Part model, mm, in its own coordinate system. A direction names the side the tool comes from. Give positions to 0.01 mm unless a question says otherwise; leave off trailing zeros. Loops run counter-clockwise (first coordinate to the right, second up) from the corner with the lowest first, then second, coordinate; pieces in that order, holes last. Notation, with made-up numbers: M 54.5,-12.75 L 113.5,-12.75 A21 cw 113.5,-5.75 Z; hole C -4,80.5 d11. An arc over 180 degrees is marked long. Put each result on its own line as item: value. Start each with the question number.
```python
from build123d import *

# Parameters (mm, degrees)
F0_W     = 15.6
F0_H     = 9.6
F1_DEPTH = 7.8
F2_R     = 2.45
F2_R_2   = 1.65
F3_DEPTH = 1.7
F5_DEPTH = 2


# Not quite as in the source:
# - a feature names something its author has since deleted; it is built from what else it names


with BuildPart() as f1:
    # F0 (on Front) → F1 (new body)
    with BuildSketch(Plane.XZ):
        with Locations((7.5497636572, 4.7150965011)):
            Rectangle(F0_W, F0_H)
        with BuildLine():
            Line((10.5497636572, 6.6150965011), (10.5497636572, 5.6150965011))
            Line((10.5497636572, 5.6150965011), (10.5497636572, 4.6150965011))
            Line((10.5497636572, 4.6150965011), (10.3781907819, 4.6150965011))
            ThreePointArc((10.3781907819, 4.6150965011), (9.6710840007, 3.4937761575), (8.5497636572, 2.7866693764))
            Line((8.5497636572, 2.7866693764), (8.5497636572, 2.6150965011))
            Line((8.5497636572, 2.6150965011), (7.5497636572, 2.6150965011))
            Line((7.5497636572, 2.6150965011), (6.5497636572, 2.6150965011))
            Line((6.5497636572, 2.6150965011), (6.5497636572, 2.7866693764))
            ThreePointArc((6.5497636572, 2.7866693764), (5.4284433136, 3.4937761575), (4.7213365324, 4.6150965011))
            Line((4.7213365324, 4.6150965011), (4.5497636572, 4.6150965011))
            Line((4.5497636572, 4.6150965011), (4.5497636572, 5.6150965067))
            Line((4.5497636572, 5.6150965067), (4.5497636572, 6.6150965011))
            Line((4.5497636572, 6.6150965011), (4.7213365324, 6.6150965011))
            ThreePointArc((4.7213365324, 6.6150965011), (5.4284433136, 7.7364168447), (6.5497636572, 8.4435236258))
            Line((6.5497636572, 8.4435236258), (6.5497636572, 8.6150965011))
            Line((6.5497636572, 8.6150965011), (7.5497636572, 8.6150965011))
            Line((7.5497636572, 8.6150965011), (8.5497636572, 8.6150965011))
            Line((8.5497636572, 8.6150965011), (8.5497636572, 8.4435236258))
            ThreePointArc((8.5497636572, 8.4435236258), (9.6710840007, 7.7364168447), (10.3781907819, 6.6150965011))
            Line((10.3781907819, 6.6150965011), (10.5497636572, 6.6150965011))
        make_face(mode=Mode.SUBTRACT)
        with BuildLine():
            ThreePointArc((8.5497636572, 2.7866693764), (9.6710840007, 3.4937761575), (10.3781907819, 4.6150965011))
            Line((10.3781907819, 4.6150965011), (8.5497636572, 4.6150965011))
            Line((8.5497636572, 4.6150965011), (8.5497636572, 2.7866693764))
        make_face()
        with BuildLine():
            Line((8.5497636572, 6.6150965011), (10.3781907819, 6.6150965011))
            ThreePointArc((10.3781907819, 6.6150965011), (9.6710840007, 7.7364168447), (8.5497636572, 8.4435236258))
            Line((8.5497636572, 8.4435236258), (8.5497636572, 6.6150965011))
        make_face()
        with BuildLine():
            Line((4.7213365324, 6.6150965011), (6.5497636572, 6.6150965011))
            Line((6.5497636572, 6.6150965011), (6.5497636572, 8.4435236258))
            ThreePointArc((6.5497636572, 8.4435236258), (5.4284433136, 7.7364168447), (4.7213365324, 6.6150965011))
        make_face()
        with BuildLine():
            Line((6.5497636572, 2.7866693764), (6.5497636572, 4.6150965011))
            Line((6.5497636572, 4.6150965011), (4.7213365324, 4.6150965011))
            ThreePointArc((4.7213365324, 4.6150965011), (5.4284433136, 3.4937761575), (6.5497636572, 2.7866693764))
        make_face()
        with BuildLine():
            Line((10.5497636572, 4.6150965011), (10.5497636572, 5.6150965011))
            ThreePointArc((10.5497636572, 5.6150965011), (10.5065593361, 5.1077905649), (10.3781907819, 4.6150965011))
            Line((10.3781907819, 4.6150965011), (10.5497636572, 4.6150965011))
        make_face()
        with BuildLine():
            ThreePointArc((10.3781907819, 6.6150965011), (10.5065593361, 6.1224024373), (10.5497636572, 5.6150965011))
            Line((10.5497636572, 5.6150965011), (10.5497636572, 6.6150965011))
            Line((10.5497636572, 6.6150965011), (10.3781907819, 6.6150965011))
        make_face()
        with BuildLine():
            ThreePointArc((7.5497636572, 8.6150965011), (8.0570695933, 8.5718921801), (8.5497636572, 8.4435236258))
            Line((8.5497636572, 8.4435236258), (8.5497636572, 8.6150965011))
            Line((8.5497636572, 8.6150965011), (7.5497636572, 8.6150965011))
        make_face()
        with BuildLine():
            ThreePointArc((6.5497636572, 8.4435236258), (7.042457721, 8.5718921801), (7.5497636572, 8.6150965011))
            Line((7.5497636572, 8.6150965011), (6.5497636572, 8.6150965011))
            Line((6.5497636572, 8.6150965011), (6.5497636572, 8.4435236258))
        make_face()
        with BuildLine():
            ThreePointArc((4.5497636572, 5.6150965067), (4.5929679787, 6.12240244), (4.7213365324, 6.6150965011))
            Line((4.7213365324, 6.6150965011), (4.5497636572, 6.6150965011))
            Line((4.5497636572, 6.6150965011), (4.5497636572, 5.6150965067))
        make_face()
        with BuildLine():
            Line((4.5497636572, 4.6150965011), (4.7213365324, 4.6150965011))
            ThreePointArc((4.7213365324, 4.6150965011), (4.5929679777, 5.1077905677), (4.5497636572, 5.6150965067))
            Line((4.5497636572, 5.6150965067), (4.5497636572, 4.6150965011))
        make_face()
        with BuildLine():
            Line((6.5497636572, 2.6150965011), (7.5497636572, 2.6150965011))
            ThreePointArc((7.5497636572, 2.6150965011), (7.042457721, 2.6583008221), (6.5497636572, 2.7866693764))
            Line((6.5497636572, 2.7866693764), (6.5497636572, 2.6150965011))
        make_face()
        with BuildLine():
            Line((8.5497636572, 2.6150965011), (8.5497636572, 2.7866693764))
            ThreePointArc((8.5497636572, 2.7866693764), (8.0570695933, 2.6583008221), (7.5497636572, 2.6150965011))
            Line((7.5497636572, 2.6150965011), (8.5497636572, 2.6150965011))
        make_face()
    extrude(amount=F1_DEPTH)

    # F2 (on face) → F3 (join)
    with BuildSketch(Plane.XY.offset(9.5150965011)):
        with Locations((3.7997636572, -3.9)):
            Circle(F2_R)
        with Locations((3.7997636572, -3.9)):
            Circle(F2_R_2, mode=Mode.SUBTRACT)
        with Locations((11.2997636572, -3.9)):
            Circle(F2_R)
        with Locations((11.2997636572, -3.9)):
            Circle(F2_R_2, mode=Mode.SUBTRACT)
    extrude(amount=F3_DEPTH)

    # F4 (on face) → F5 (cut)
    with BuildSketch(Plane(origin=(0, 0, -0.0849034989), x_dir=(1, 0, 0), z_dir=(0, 0, -1))):
        Polygon((1.3497636572, 6.2), (1.3497636572, 3.9), (1.3497636572, 1.6), (7.5497636572, 1.6), (13.7497636572, 1.6), (13.7497636572, 3.9), (13.7497636572, 6.2), (7.5497636572, 6.2), align=None)
    extrude(amount=-F5_DEPTH, mode=Mode.SUBTRACT)


solid = f1.part
```
1) Which spindle directions (+Z, -Z, +X, -X, +Y, -Y) get a long thin tool onto all of the face, cutting with end or side? Do faces 4 (the flat face through (15.35, -4, 5)), 5 (the flat face through (11, -4, 9.515)), 6 (the flat face through (7, -4, 1.915)), 7 (the flat face through (9, -4, 6.615)). Say none if no direction does.
2) Mould opens along Y. For faces 1 (the flat face through (6.55, -4, 4)), 2 (the flat face through (4, -4, 9.515)), 3 (the flat face through (9, -7.8, 4)) say: +Y half, -Y half, draft (parallel to the pull), parting line (faces both ways), or undercut.
3) Wall check: L1, parallel to X at y = -7.5, z = 8; L2, parallel to Z at x = 6, y = -5.75; L3, parallel to Z at x = 5.75, y = -1. Give the ranges that are in metal, low to high.
4) Band-saw the part on A-A on z = 7. Give the cut face in (x, y), then the cut area to 3 significant figures.
5) Band-saw the part on B-B on y = -1. Give the cut face in (x, z), then the cut area to 3 significant figures.
6) Band-saw the part on D-D on x = 6. Give the cut face in (y, z), then the cut area to 3 significant figures.
7) Pin check, flat tips, straight feed: pin 1 Ø2 at (x, z) = (7.5, 3.5) entering from +Y; pin 2 Ø1.5 at (x, y) = (5.5, -5) entering from -Z; pin 3 Ø1 at (x, y) = (12, -4) entering from +Z. Stop position of each tip, or through.
8) Band-saw the part on C-C on z = 10.75. Give the cut face in (x, y), then the cut area to 3 significant figures.
Evaluation:
1. face 4: +Z, -Z, +X, +Y, -Y
1. face 5: +Z
1. face 6: -Z
1. face 7: +Y, -Y
2. face 1: draft
2. face 2: undercut
2. face 3: -Y half
3. L1: -0.25 to 6.55, 8.55 to 15.35
3. L2: 1.92 to 4.62, 6.62 to 9.52
3. L3: -0.08 to 4.62, 6.62 to 9.52
4. outline: M -0.25,-7.8 L 6.55,-7.8 L 6.55,0 L -0.25,0 Z; M 8.55,-7.8 L 15.35,-7.8 L 15.35,0 L 8.55,0 Z
4. area: 106 mm2
5. outline: M -0.25,-0.08 L 15.35,-0.08 L 15.35,9.52 L -0.25,9.52 Z; hole M 4.72,4.62 L 6.55,4.62 L 6.55,2.79 A3 ccw 8.55,2.79 L 8.55,4.62 L 10.38,4.62 A3 ccw 10.38,6.62 L 8.55,6.62 L 8.55,8.44 A3 ccw 6.55,8.44 L 6.55,6.62 L 4.72,6.62 A3 ccw Z
5. area: 130 mm2
6. outline: M -7.8,-0.08 L -6.2,-0.08 L -6.2,1.92 L -1.6,1.92 L -1.6,-0.08 L 0,-0.08 L 0,4.62 L -7.8,4.62 Z; M -7.8,6.62 L 0,6.62 L 0,9.52 L -2.82,9.52 L -2.82,11.22 L -4.98,11.22 L -4.98,9.52 L -7.8,9.52 Z
6. area: 53.7 mm2
7. pin 1: y = 0
7. pin 2: z = 1.92
7. pin 3: z = 9.52
8. outline: C 3.8,-3.9 d4.9; C 11.3,-3.9 d4.9; hole C 3.8,-3.9 d3.3; hole C 11.3,-3.9 d3.3
8. area: 20.6 mm2
